Build history of the part. All positions in model axes, mm. A direction names the side the tool comes from. Give positions to 0.01 mm unless a question says otherwise; leave off trailing zeros. Loops run counter-clockwise (first coordinate to the right, second up) from the corner with the lowest first, then second, coordinate; pieces in that order, holes last. Notation, with made-up numbers: M 84.25,64 L 90.25,64 A14 cw 90.25,83 Z; hole C 67,16.25 d7. An arc over 180 degrees is marked long. Answer in a Markdown table with one row per item. Add a question column.
```python
from build123d import *

# Parameters (mm, degrees)
SZKIC1_W                    = 56.4
SZKIC1_H                    = 56.4
DODANIE_WYCI_GNI_CIE1_DEPTH = 105
SZKIC2_R                    = 4
DODANIE_WYCI_GNI_CIE2_DEPTH = 20
SZKIC3_W                    = 8.2
SZKIC3_H                    = 8.2
WYTNIJ_WYCI_GNI_CIE1_DEPTH  = 100
ZAOKR_GLENIE1_R             = 2
SFAZOWANIE1_SIZE            = 2
OTW_R_POD_RUB_M51_D         = 5.5
OTW_R_POD_RUB_M51_DEPTH     = 11
OTW_R_POD_RUB_M51_TIP       = 1.652366702
SFAZOWANIE2_SIZE            = 1


with BuildPart() as part:
    # Szkic1 → Dodanie-wyciągnięcie1 (new body)
    with BuildSketch(Plane.XY):
        Rectangle(SZKIC1_W, SZKIC1_H)
    extrude(amount=DODANIE_WYCI_GNI_CIE1_DEPTH)

    # Szkic2 → Dodanie-wyciągnięcie2 (add)
    with BuildSketch(Plane(origin=(0, 0, 0), x_dir=(-1, 0, 0), z_dir=(0, 0, -1))):
        with Locations(Location((0, 0, 0), (0, 0, 180))):
            Circle(SZKIC2_R)
    extrude(amount=DODANIE_WYCI_GNI_CIE2_DEPTH)

    # Szkic3 → Wytnij-wyciągnięcie1 (cut)
    with BuildSketch(Plane.XY.offset(105)):
        with Locations((-24.1, 24.1)):
            Rectangle(SZKIC3_W, SZKIC3_H)
        with Locations((24.1, 24.1)):
            Rectangle(SZKIC3_W, SZKIC3_H)
        with Locations((24.1, -24.1)):
            Rectangle(SZKIC3_W, SZKIC3_H)
        with Locations((-24.1, -24.1)):
            Rectangle(SZKIC3_W, SZKIC3_H)
    extrude(amount=-WYTNIJ_WYCI_GNI_CIE1_DEPTH, mode=Mode.SUBTRACT)

    # Zaokrąglenie1
    zaokr_glenie1_edges = [part.edges().sort_by_distance(p)[0] for p in [
        (-20, -28.2, 55),
        (-28.2, -20, 55),
        (-20, -20, 55),
        (28.2, -20, 55),
        (20, -28.2, 55),
        (20, -20, 55),
        (20, 28.2, 55),
        (28.2, 20, 55),
        (20, 20, 55),
        (-28.2, 20, 55),
        (-20, 28.2, 55),
        (-20, 20, 55),
    ]]
    fillet(zaokr_glenie1_edges, radius=ZAOKR_GLENIE1_R)

    # Sfazowanie1
    sfazowanie1_edges = [part.edges().sort_by_distance(p)[0] for p in [
        (-20.585786438, -20.585786438, 105),
        (20.585786438, -20.585786438, 105),
        (20.585786438, 20.585786438, 105),
        (-20.585786438, 20.585786438, 105),
        (28.2, -28.2, 2.5),
        (-28.2, -28.2, 2.5),
        (-28.2, 28.2, 2.5),
        (28.2, 28.2, 2.5),
        (-20, -24.1, 105),
        (0, -28.2, 105),
        (20, -24.1, 105),
        (24.1, -20, 105),
        (28.2, 0, 105),
        (24.1, 20, 105),
        (20, 24.1, 105),
        (0, 28.2, 105),
        (-20, 24.1, 105),
        (-24.1, 20, 105),
        (-28.2, 0, 105),
        (-24.1, -20, 105),
        (-27.614213562, 19.414213562, 105),
        (-19.414213562, 27.614213562, 105),
        (19.414213562, 27.614213562, 105),
        (27.614213562, 19.414213562, 105),
        (27.614213562, -19.414213562, 105),
        (19.414213562, -27.614213562, 105),
        (-27.614213562, -19.414213562, 105),
        (-19.414213562, -27.614213562, 105),
    ]]
    chamfer(sfazowanie1_edges, length=SFAZOWANIE1_SIZE)

    # Otwór pod śrubę M51
    with Locations(Plane(origin=(0, 0, 0), x_dir=(-1, 0, 0), z_dir=(0, 0, -1))):
        with Locations((-23.57, 23.57), (23.57, 23.57), (23.57, -23.57), (-23.57, -23.57)):
            Hole(OTW_R_POD_RUB_M51_D / 2, depth=OTW_R_POD_RUB_M51_DEPTH)
            with Locations((0, 0, -(OTW_R_POD_RUB_M51_DEPTH + OTW_R_POD_RUB_M51_TIP / 2))):  # 118° drill point
                Cone(0, OTW_R_POD_RUB_M51_D / 2, OTW_R_POD_RUB_M51_TIP, mode=Mode.SUBTRACT)

    # Sfazowanie2
    sfazowanie2_edges = [part.edges().sort_by_distance(p)[0] for p in [
        (-4, 0, -20),
    ]]
    chamfer(sfazowanie2_edges, length=SFAZOWANIE2_SIZE)


solid = part.part
```
(1) Pull direction X, two halves, no side cores. Call faces 6 (the flat face through (20, -24, 55)), 7 (the cylindrical face through (22.974, 20.885, 2.535)), 8 (the flat face through (-7, 0, 0)): +X half, -X half, draft (parallel to the pull), parting line (faces both ways), or undercut.
(2) Pin check, flat tips, straight feed: pin 1 (1.3 mm diameter, centred on x = 24.5, z = 39.5, fed in from -Y); pin 2 (5 mm diameter, centred on x = -23.5, y = 25.5, fed in from +Z); pin 3 (9 mm diameter, centred on x = -23.57, y = 23.57, fed in from -Z). Stop position of each tip, or through.
(3) Tool access for faces 1 (the flat face through (24, 20, 55)), 2 (the flat face through (24, -20, 55)), 3 (the cylindrical face through (-0.867, 3.905, -9.367)), 4 (the flat face through (-20, -24, 55)), 5 (the flat face through (-20, 24, 55)): list every direction of +Z, -Z, +X, -X, +Y, -Y with a clear straight run to the whole face (end or side of a thin tool).
(4) Slice it at A-A, the plane y = 23.57. Give the cut face in (x, z), then the cut area to 3 significant figures.
(5) Wall check: line 1 (Y direction, x = -23.57, z = 3.5); line 2 (X direction, y = 23, z = 1); line 3 (Z direction, x = 16, y = 15.5). Give the ranges that are in metal, low to high.
(6) Slice it at C-C, the plane z = 31. Give the cut face in (x, y), then the cut area to 3 significant figures.
(7) Slice it at B-B, the plane x = 0. Give the cut face in (y, z).
Solution:
| question | item | result |
|---|---|---|
| 1 | face 6 | +X half |
| 1 | face 7 | undercut |
| 1 | face 8 | draft |
| 2 | pin 1 | y = -20 |
| 2 | pin 2 | z = 5 |
| 2 | pin 3 | z = 0 |
| 3 | face 1 | +Z, +X, +Y |
| 3 | face 2 | +Z, +X, -Y |
| 3 | face 3 | -Z |
| 3 | face 4 | +Z, -X, -Y |
| 3 | face 5 | +Z, -X, +Y |
| 4 | outline | M -28.2,0 L -26.32,0 L -26.32,5 L -28.2,5 Z; M -20.82,0 L 20.82,0 L 20.82,5 L 20,5 L 20,103 L 18,105 L -18,105 L -20,103 L -20,5 L -20.82,5 Z; M 26.32,0 L 28.2,0 L 28.2,5 L 26.32,5 Z |
| 4 | area | 4,220 mm^2 |
| 5 | line 1 | -28.2 to -26.32, -20.82 to 20.82, 26.32 to 28.2 |
| 5 | line 2 | -28.2 to -26.26, -20.88 to 20.88, 26.26 to 28.2 |
| 5 | line 3 | 0 to 105 |
| 6 | outline | M -28.2,-18 A2 ccw -26.2,-20 L -22,-20 A2 cw -20,-22 L -20,-26.2 A2 ccw -18,-28.2 L 18,-28.2 A2 ccw 20,-26.2 L 20,-22 A2 cw 22,-20 L 26.2,-20 A2 ccw 28.2,-18 L 28.2,18 A2 ccw 26.2,20 L 22,20 A2 cw 20,22 L 20,26.2 A2 ccw 18,28.2 L -18,28.2 A2 ccw -20,26.2 L -20,22 A2 cw -22,20 L -26.2,20 A2 ccw -28.2,18 Z |
| 6 | area | 2,910 mm^2 |
| 7 | outline | M -28.2,0 L -4,0 L -4,-19 L -3,-20 L 3,-20 L 4,-19 L 4,0 L 28.2,0 L 28.2,103 L 26.2,105 L -26.2,105 L -28.2,103 Z |
